from build123d import *

# Parameters (mm, degrees)
BOSS_EXTRUDE1_DEPTH     = 8
CUT_EXTRUDE1_DEPTH      = 72.444471445
CUT_EXTRUDE1_DEPTH_BACK = 72.444471445
SKETCH2_R               = 3.1
FILLET1_R               = 6
CUT_EXTRUDE2_DEPTH      = 72.444471445
CUT_EXTRUDE2_DEPTH_BACK = 6
SKETCH3_R               = 5.7


with BuildPart() as part:
    # Sketch1 → Boss-Extrude1 (new body)
    with BuildSketch(Plane(origin=(0, 0, 0), x_dir=(1, 0, 0), z_dir=(0, 1, 0))):
        Polygon((-31.75, 0), (31.75, 0), (31.75, 25.4), (12.7, 63.5), (-12.7, 63.5), (-31.75, 25.4), align=None)
    extrude(amount=BOSS_EXTRUDE1_DEPTH)

    # Sketch2 → Cut-Extrude1 (cut, two sides: drawn at the far end of the back side and taken through both)
    with BuildSketch(Plane(origin=(0, 8, 0), x_dir=(1, 0, 0), z_dir=(0, 1, 0)).offset(-CUT_EXTRUDE1_DEPTH_BACK)):
        with Locations(Location((0, 50.8, 0), (0, 0, 270))):
            Circle(SKETCH2_R)
        with Locations(Location((-19.05, 12.7, 0), (0, 0, 270))):
            Circle(SKETCH2_R)
        with Locations(Location((19.05, 12.7, 0), (0, 0, 270))):
            Circle(SKETCH2_R)
    extrude(amount=CUT_EXTRUDE1_DEPTH + CUT_EXTRUDE1_DEPTH_BACK, mode=Mode.SUBTRACT)

    # Fillet1
    fillet1_edges = [part.edges().sort_by_distance(p)[0] for p in [
        (31.75, 4, 0),
        (-31.75, 4, 0),
        (-31.75, 4, -25.4),
        (-12.7, 4, -63.5),
        (12.7, 4, -63.5),
        (31.75, 4, -25.4),
    ]]
    fillet(fillet1_edges, radius=FILLET1_R)

    # Sketch3 → Cut-Extrude2 (cut, two sides: drawn at the far end of the back side and taken through both)
    with BuildSketch(Plane(origin=(0, 8, 0), x_dir=(1, 0, 0), z_dir=(0, 1, 0)).offset(-CUT_EXTRUDE2_DEPTH_BACK)):
        with Locations(Location((-19.05, 12.7, 0), (0, 0, 90))):
            Circle(SKETCH3_R)
        with Locations(Location((19.05, 12.7, 0), (0, 0, 90))):
            Circle(SKETCH3_R)
        Polygon((5.888972746, 50.8), (2.944486373, 55.9), (-2.944486373, 55.9), (-5.888972746, 50.8), (-2.944486373, 45.7), (2.944486373, 45.7), align=None)
    extrude(amount=CUT_EXTRUDE2_DEPTH + CUT_EXTRUDE2_DEPTH_BACK, mode=Mode.SUBTRACT)


solid = part.part
Build history of the part. All positions in model axes, mm. A direction names the side the tool comes from. Round coordinates to 2 decimals unless told otherwise and drop trailing zeros. Loops run counter-clockwise (first coordinate to the right, second up) from the corner with the lowest first, then second, coordinate; pieces in that order, holes last. Notation, with made-up numbers: (-14.5, 0.25) -> (-6.5, 0.25) arc R18 ccw to (-6.5, 11.25) -> close; hole circle Ø10 at (57.25, 68). An arc over 180 degrees is marked (long way). One line per item, written item: value. Start each with the question number.
Q1. 3-axis set-ups, long thin cutter, end or side, ignore diameter. For faces 1 (the face through (3, 2, -53)), 2 (the face through (0, 4, 0)): which of +Z, -Z, +X, -X, +Y, -Y reach the whole face in a straight line?
Q2. Cut at A-A on z = -12.7. List the corners of the cut face in (x, y), plus the area to 3 significant figures.
Q3. Drop flat-ended pins along their axis: pin 1 Ø3.5 at (x, z) = (19, -15) entering from +Y; pin 2 Ø2 at (y, z) = (4, -31) entering from -X. Give the stop position or say it passes through.
Q4. Two-plate mould, pull along X, no slides. Class faces 3 (the face through (-13.486, 4.958, -11.464)), 4 (the face through (-29.946, 4.056, -1.711)), 5 (the face through (22, 2, -15)), 6 (the face through (22.855, 3.944, -43.19)): released by +X, released by -X, zero draft, split by the parting line, or undercut.
Q5. Cut at B-B on y = 6. List the corners of the cut face in (x, z), plus the area to 3 significant figures.
Q6. Cut at C-C on x = -19.05. List the corners of the cut face in (y, z), plus the area to 3 significant figures.
Q7. Cut at D-D on x = 0. List the corners of the cut face in (y, z).
Q8. Probe line 1 along X through (y, z) = (6.7, -12.7); line 2 along X through (y, z) = (1, -12.7); line 3 along Z through (x, y) = (-19.05, 6.3). List the from-to ranges inside material, lowest first.
Computed:
1. face 1: +Y
1. face 2: +Z, +X, -X, +Y, -Y
2. outline: (-31.75, 0) -> (-22.15, 0) -> (-22.15, 2) -> (-24.75, 2) -> (-24.75, 8) -> (-31.75, 8) -> close; (-15.95, 0) -> (15.95, 0) -> (15.95, 2) -> (13.35, 2) -> (13.35, 8) -> (-13.35, 8) -> (-13.35, 2) -> (-15.95, 2) -> close; (22.15, 0) -> (31.75, 0) -> (31.75, 8) -> (24.75, 8) -> (24.75, 2) -> (22.15, 2) -> close
2. area: 346 mm²
3. pin 1: y = 2
3. pin 2: x = -29.45
4. face 3: undercut
4. face 4: released by -X
4. face 5: undercut
4. face 6: released by +X
5. outline: (-31.75, -23.98) arc R6 ccw to (-31.12, -26.67) -> (-14.36, -60.18) arc R6 ccw to (-8.99, -63.5) -> (8.99, -63.5) arc R6 ccw to (14.36, -60.18) -> (31.12, -26.67) arc R6 ccw to (31.75, -23.98) -> (31.75, -6) arc R6 ccw to (25.75, 0) -> (-25.75, 0) arc R6 ccw to (-31.75, -6) -> close; hole circle Ø11.4 at (-19.05, -12.7); hole (-5.89, -50.8) -> (-2.94, -55.9) -> (2.94, -55.9) -> (5.89, -50.8) -> (2.94, -45.7) -> (-2.94, -45.7) -> close; hole circle Ø11.4 at (19.05, -12.7)
5. area: 2,990 mm²
6. outline: (0, -50.8) -> (8, -50.8) -> (8, -18.4) -> (2, -18.4) -> (2, -15.8) -> (0, -15.8) -> close; (0, -9.6) -> (2, -9.6) -> (2, -7) -> (8, -7) -> (8, 0) -> (0, 0) -> close
6. area: 326 mm²
7. outline: (0, -63.5) -> (8, -63.5) -> (8, -55.9) -> (2, -55.9) -> (2, -53.9) -> (0, -53.9) -> close; (0, -47.7) -> (2, -47.7) -> (2, -45.7) -> (8, -45.7) -> (8, 0) -> (0, 0) -> close
8. line 1: -31.75 to -24.75, -13.35 to 13.35, 24.75 to 31.75
8. line 2: -31.75 to -22.15, -15.95 to 15.95, 22.15 to 31.75
8. line 3: -50.8 to -18.4, -7 to 0
